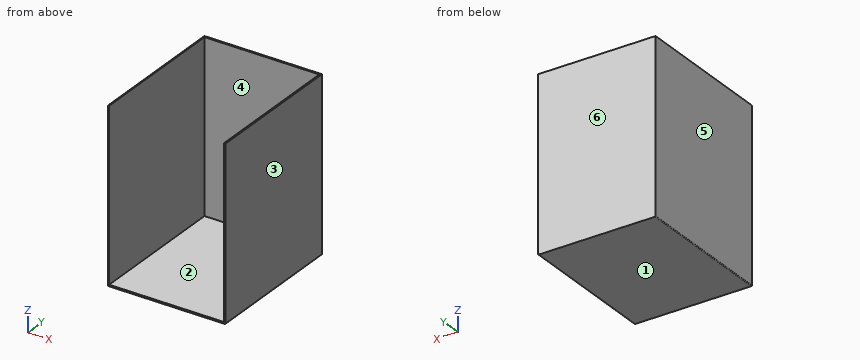
from build123d import *

# Parameters (mm, degrees)
F1_DEPTH = 426
F2_W     = 295
F2_H     = 360
F3_DEPTH = 4
F4_R     = 2


# Not quite as in the source:
# - a feature names something its author has since deleted; it is built from what else it names


with BuildPart() as f1:
    # F0 (on Top) → F1 (new body)
    with BuildSketch(Plane.XY):
        Polygon((-4, -360), (0, -360), (0, 0), (-295, 0), (-295, -360), (-292.1838745495, -360), (-292.1838745495, -4), (-4, -4), align=None)
    extrude(amount=F1_DEPTH)

    # F2 (on Top) → F3 (join)
    with BuildSketch(Plane.XY):
        with Locations((-147.5, -180)):
            Rectangle(F2_W, F2_H)
    extrude(amount=-F3_DEPTH)

    # F4
    f4_edges = [f1.edges().sort_by_distance(p)[0] for p in [
        (-295, -180, -4),
        (0, -180, -4),
    ]]
    fillet(f4_edges, radius=F4_R)


solid = f1.part
Input: part model. Units: mm. Frame: model coordinates. Face numbers are marked on the shaded views. A direction names the side the tool comes from. Give positions to 0.01 mm unless a question says otherwise; leave off trailing zeros. Loops run counter-clockwise (first coordinate to the right, second up) from the corner with the lowest first, then second, coordinate; pieces in that order, holes last. Notation, with made-up numbers: M 29.5,-22 L 82.5,-22 A21 cw 82.5,6 Z; hole C 66,34 d1. An arc over 180 degrees is marked long. Use one line per item in the form item = value.
1. First-contact query: pin 1 (12 mm diameter, centred on x = -50, z = 60, fed in from -Y); pin 2 (5 mm diameter, centred on x = -149.5, z = 354, fed in from +Y); pin 3 (8 mm diameter, centred on x = -240.5, y = -321, fed in from +Z). Flat tips, straight axial feed; report the tip coordinate or a pass-through.
Numbers:
pin_1 = -4
pin_2 = 0
pin_3 = 0
2. Section query A-A, the plane z = 59. Return the cut outline in (x, y), and give its area (3 significant figures).
Numbers:
outline = M -295,-360 L -292.18,-360 L -292.18,-4 L -4,-4 L -4,-360 L 0,-360 L 0,0 L -295,0 Z
area = 3,610 mm²
3. Pull-direction query (X, two-part tool) for the marked faces 3, 4, 5 and 6; classes: released by +X, released by -X, zero draft, split by the parting line, or undercut.
Numbers:
face_3 = released by +X
face_4 = undercut
face_5 = released by -X
face_6 = zero draft
4. Section query C-C, the plane x = -64.5. Return the cut outline in (y, z).
Numbers:
outline = M -360,-4 L 0,-4 L 0,426 L -4,426 L -4,0 L -360,0 Z
5. Line query: L1, parallel to X at y = -181, z = 134; L2, parallel to Y at x = -126, z = 173.5. Output: solid intervals per line, ascending.
Numbers:
L1 = -295 to -292.18, -4 to 0
L2 = -4 to 0
6. Section query B-B, the plane y = -45.5. Return the cut outline in (x, z), and give its area (3 significant figures).
Numbers:
outline = M -295,-2 A2 ccw -293,-4 L -2,-4 A2 ccw 0,-2 L 0,426 L -4,426 L -4,0 L -292.18,0 L -292.18,426 L -295,426 Z
area = 4,080 mm²
7. Reachability of the marked faces 1 and 2 from +Z, -Z, +X, -X, +Y, -Y: full face, straight path, thin tool, end or side. Return the list, or none.
Numbers:
face_1 = -Z, +X, -X, +Y, -Y
face_2 = +Z, -Y
